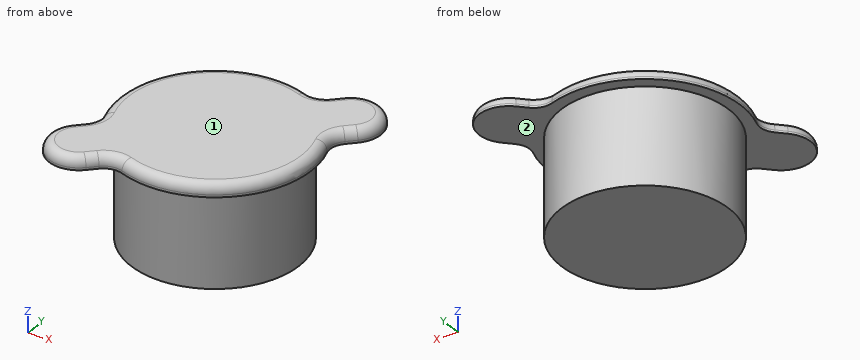
```python
from build123d import *

# Parameters (mm, degrees)
SKETCH1_R           = 22.225
BOSS_EXTRUDE1_DEPTH = 3.175
FILLET1_R           = 2.54
SKETCH1_3_R         = 22.225
BOSS_EXTRUDE2_DEPTH = 25.4


with BuildPart() as part:
    # Sketch1 → Boss-Extrude1 (new body)
    # profile 1 of 2: a face of its own
    with BuildSketch(Plane.XY):
        with BuildLine():
            Line((25.100798696, 13.875478544), (27.165274766, 15.939954615))
            ThreePointArc((27.165274766, 15.939954615), (27.165274766, 27.165274766), (15.939954615, 27.165274766))
            Line((15.939954615, 27.165274766), (13.875478544, 25.100798696))
            ThreePointArc((13.875478544, 25.100798696), (11.395117189, 23.736044101), (8.56948008, 23.910750953))
            ThreePointArc((8.56948008, 23.910750953), (-17.960512242, 17.960512242), (-23.910750953, -8.56948008))
            ThreePointArc((-23.910750953, -8.56948008), (-23.736044101, -11.395117189), (-25.100798696, -13.875478544))
            Line((-25.100798696, -13.875478544), (-27.165274766, -15.939954615))
            ThreePointArc((-27.165274766, -15.939954615), (-27.165274766, -27.165274766), (-15.939954615, -27.165274766))
            Line((-15.939954615, -27.165274766), (-13.875478544, -25.100798696))
            ThreePointArc((-13.875478544, -25.100798696), (-11.395117189, -23.736044101), (-8.56948008, -23.910750953))
            ThreePointArc((-8.56948008, -23.910750953), (17.960512242, -17.960512242), (23.910750953, 8.56948008))
            ThreePointArc((23.910750953, 8.56948008), (23.736044101, 11.395117189), (25.100798696, 13.875478544))
        make_face()
        Circle(SKETCH1_R, mode=Mode.SUBTRACT)
    # profile 2 of 2: a face of its own
    with BuildSketch(Plane.XY):
        Circle(SKETCH1_R)
    extrude(amount=BOSS_EXTRUDE1_DEPTH)

    # Fillet1
    fillet1_edges = [part.edges().sort_by_distance(p)[0] for p in [
        (27.165274766, 27.165274766, 3.175),
        (14.90771658, 26.133036731, 3.175),
        (11.395117189, 23.736044101, 3.175),
        (-17.960512242, 17.960512242, 3.175),
        (-23.736044101, -11.395117189, 3.175),
        (-26.133036731, -14.90771658, 3.175),
        (-27.165274766, -27.165274766, 3.175),
        (-14.90771658, -26.133036731, 3.175),
        (26.133036731, 14.90771658, 3.175),
        (-11.395117189, -23.736044101, 3.175),
        (17.960512242, -17.960512242, 3.175),
        (23.736044101, 11.395117189, 3.175),
    ]]
    fillet(fillet1_edges, radius=FILLET1_R)

    # Sketch1<3> → Boss-Extrude2 (add)
    with BuildSketch(Plane.XY):
        Circle(SKETCH1_3_R)
    extrude(amount=-BOSS_EXTRUDE2_DEPTH)


solid = part.part
```
CAD build for the part. Positions are in the model's coordinates, mm. Face numbers are marked on the shaded views. A direction names the side the tool comes from. Round coordinates to 2 decimals unless told otherwise and drop trailing zeros. Write each loop counter-clockwise with the first axis right and the second up, starting at its lowest first coordinate (ties: lowest second). Pieces come first, ordered by that corner, then holes.
Item 1: Band-saw the part on A-A on z = -6.75. Write the cut outline in (x, y) (3 decimals).
Filled in:
outline: circle Ø44.45 at (0, 0)
Item 2: Drop flat-ended pins along their axis: pin 1 Ø3 at (x, z) = (1, -8) entering from +Y (3 decimals); pin 2 Ø1.5 at (x, z) = (-10.5, -6.5) entering from +Y; pin 3 Ø8 at (x, z) = (-15, -7) entering from -Y. Give the stop position or say it passes through.
Filled in:
pin 1: stops at y = 22.225
pin 2: stops at y = 19.97
pin 3: stops at y = -19.31
Item 3: Tool access for the marked faces 1 and 2: list every direction of +Z, -Z, +X, -X, +Y, -Y with a clear straight run to the whole face (end or side of a thin tool).
Filled in:
face 1: +Z, +X, -X, +Y, -Y
face 2: -Z
Item 4: Drill centre lines: L1, parallel to Y at x = 20.5, z = -12.75; L2, parallel to X at y = -0.5, z = -21; L3, parallel to Z at x = 16, y = 19 (3 decimals). Where is each one in solid material? Low to high.
Filled in:
L1: y = -8.58 to 8.58
L2: x = -22.22 to 22.22
L3: z = 0 to 3.175
